Geometry check sheet. Reference: the model listing, model coordinates, mm. Round coordinates to 2 decimals unless told otherwise and drop trailing zeros. Loops run counter-clockwise (first coordinate to the right, second up) from the corner with the lowest first, then second, coordinate; pieces in that order, holes last. Notation, with made-up numbers: (49, 0) - (96, 0) arc R15 ccw to (96, 5) - close; hole circle Ø10 at (83.25, 68). An arc over 180 degrees is marked (long way). Answer in a Markdown table with one row per item. Add a question column.
```python
from build123d import *

# Parameters (mm, degrees)
SKETCH_1_R      = 1
EXTRUDE_1_DEPTH = 2


with BuildPart() as part:
    # 草图1 → 凸台-拉伸1 (new body)
    with BuildSketch(Plane.XY):
        Polygon((-27, 4), (27, 4), (27, 2), (30, 2), (30, 3.5), (32, 3.5), (32, 2), (36, 2), (36, 4), (38, 4), (38, -4), (36, -4), (36, -2), (32, -2), (32, -3.5), (30, -3.5), (30, -2), (27, -2), (27, -4), (-27, -4), (-27, -2), (-30, -2), (-30, -3.5), (-32, -3.5), (-32, -2), (-36, -2), (-36, -4), (-38, -4), (-38, 4), (-36, 4), (-36, 2), (-32, 2), (-32, 3.5), (-30, 3.5), (-30, 2), (-27, 2), align=None)
        Circle(SKETCH_1_R, mode=Mode.SUBTRACT)
        with Locations((5, 0)):
            Circle(SKETCH_1_R, mode=Mode.SUBTRACT)
        with Locations((10, 0)):
            Circle(SKETCH_1_R, mode=Mode.SUBTRACT)
        with Locations((15, 0)):
            Circle(SKETCH_1_R, mode=Mode.SUBTRACT)
        with Locations((20, 0)):
            Circle(SKETCH_1_R, mode=Mode.SUBTRACT)
        with Locations((-5, 0)):
            Circle(SKETCH_1_R, mode=Mode.SUBTRACT)
        with Locations((-10, 0)):
            Circle(SKETCH_1_R, mode=Mode.SUBTRACT)
        with Locations((-15, 0)):
            Circle(SKETCH_1_R, mode=Mode.SUBTRACT)
        with Locations((-20, 0)):
            Circle(SKETCH_1_R, mode=Mode.SUBTRACT)
    extrude(amount=EXTRUDE_1_DEPTH)


solid = part.part
```
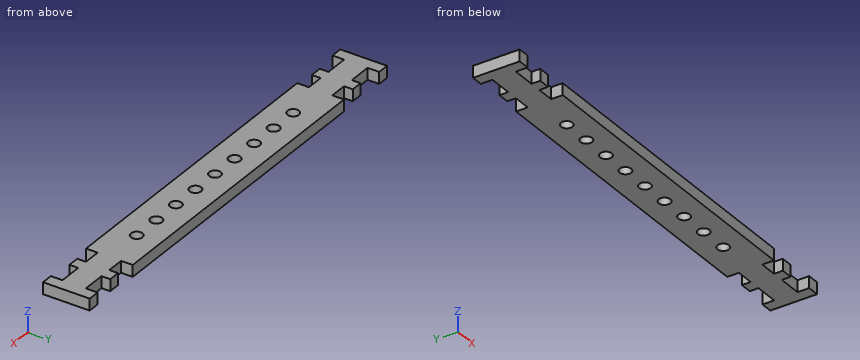
Q1. Cross-section at C-C, the plane z = 0.75. State how many separate pieces and enclosed holes the cut face has, plus the area to 3 significant figures.
Q2. Depth check by flat-ended pin: P1, Ø1, axis at x = -28, z = 1, coming from the -Y side. Enter the tip coordinate at first touch or a pass-through.
Q3. Cross-section at B-B, the plane y = 2.75. Enter the section's corners in (x, z), plus the area to 3 significant figures.
Q4. Cross-section at A-A, the plane x = 0. Enter the section's corners in (y, z).
Q5. Scan lines: line 1 (X direction, y = 3.25, z = 1.3); line 2 (Y direction, x = 20, z = 1.2); line 3 (X direction, y = 3.75, z = 0.4). Record each from-to range of solid material in increasing order. Write a range as from..to.
Check sheet entries:
| question | item | result |
|---|---|---|
| 1 | separate pieces | 1 |
| 1 | enclosed holes | 9 |
| 1 | area | 520 mm² |
| 2 | P1 | y = -2 |
| 3 | outline | (-38, 0) - (-36, 0) - (-36, 2) - (-38, 2) - close; (-32, 0) - (-30, 0) - (-30, 2) - (-32, 2) - close; (-27, 0) - (27, 0) - (27, 2) - (-27, 2) - close; (30, 0) - (32, 0) - (32, 2) - (30, 2) - close; (36, 0) - (38, 0) - (38, 2) - (36, 2) - close |
| 3 | area | 124 mm² |
| 4 | outline | (-4, 0) - (-1, 0) - (-1, 2) - (-4, 2) - close; (1, 0) - (4, 0) - (4, 2) - (1, 2) - close |
| 5 | line 1 | -38..-36, -32..-30, -27..27, 30..32, 36..38 |
| 5 | line 2 | -4..-1, 1..4 |
| 5 | line 3 | -38..-36, -27..27, 36..38 |
